Here's how the part is built. I have some questions about the finished solid (model axes, mm). A direction names the side the tool comes from. Give positions to 0.01 mm unless a question says otherwise; leave off trailing zeros. Write each loop counter-clockwise with the first axis right and the second up, starting at its lowest first coordinate (ties: lowest second). Pieces come first, ordered by that corner, then holes. Notation, with made-up numbers: M 75.5,-31.75 L 101.5,-31.75 A13 ccw 101.5,-18.75 Z; hole C 81.25,5 d11. An arc over 180 degrees is marked long. Use one line per item in the form item = value. Start each with the question number.
from build123d import *
from build123d.topology import SkipClean

# Parameters (mm, degrees)
SKETCH1_R                = 1.25
BOSS_EXTRUDE1_DEPTH      = 11
BOSS_EXTRUDE2_DEPTH      = 1.25
BOSS_EXTRUDE2_DEPTH_BACK = 1.25
SKETCH2_R                = 1.75
SKETCH3_R                = 0.75
CUT_EXTRUDE2_DEPTH       = 3


with BuildPart() as part:
    # Sketch1 → Boss-Extrude1 (new body)
    with BuildSketch(Plane(origin=(0, 0, 0), x_dir=(1, 0, 0), z_dir=(0, 1, 0))):
        with Locations(Location((0, 0, 0), (0, 0, 270))):
            Circle(SKETCH1_R)
    extrude(amount=BOSS_EXTRUDE1_DEPTH)

    # Sketch2 → Boss-Extrude2 (add, two sides: drawn at the far end of the back side and taken through both)
    with SkipClean():  # the faces are left unmerged after this step: merging them gives an invalid solid
        with BuildSketch(Plane(origin=(0, 0, 0), x_dir=(0, 0, -1), z_dir=(1, 0, 0)).offset(-BOSS_EXTRUDE2_DEPTH_BACK)):
            Circle(SKETCH2_R)
        extrude(amount=BOSS_EXTRUDE2_DEPTH + BOSS_EXTRUDE2_DEPTH_BACK)

    # Sketch3 → Cut-Extrude2 (cut)
    with SkipClean():  # the faces are left unmerged after this step: merging them gives an invalid solid
        with BuildSketch(Plane(origin=(1.25, 0, 0), x_dir=(0, 0, -1), z_dir=(1, 0, 0))):
            Circle(SKETCH3_R)
        extrude(amount=-CUT_EXTRUDE2_DEPTH, mode=Mode.SUBTRACT)


solid = part.part
1) Suppose I cut it at D-D, the plane y = 7.75. List the corners of the cut face in (x, z) for me, and give its area (3 significant figures).
2) Suppose I cut it at C-C, the plane z = -1.4. List the corners of the cut face in (x, y) for me.
3) Suppose I cut it at A-A, the plane x = 0. List the corners of the cut face in (y, z) for me.
4) Please list where these lines run through material, in increasing order: line 1 (Z direction, x = -0.05, y = 0); line 2 (Y direction, x = 0, z = 0); line 3 (Z direction, x = -1, y = 7).
5) Thinking about a two-plate mould opening in Y: for faces 1 (the face through (0, 11, 0)), 2 (the face through (1.25, -1, 0)), 3 (the face through (0.02, 0.03, 0.75)), which applies, released by +Y, released by -Y, zero draft, split by the parting line, or undercut?
6) Suppose I cut it at B-B, the plane y = 0.5. List the corners of the cut face in (x, z) for me, and give its area (3 significant figures).
7) On a 3-axis mill with a long thin cutter (end or side, diameter ignored), from which of +Z, -Z, +X, -X, +Y, -Y can I reach the whole of each face in a straight line? I mean faces 4 (the face through (-1.25, -1, 0)), 5 (the face through (0.38, 6.04, 1.19)). Say none if no direction works.
8) Will this pin go through, and if not, where does the flat tip stop? P1, Ø1, axis at x = 0.5, y = 3.5, coming from the -Z side.
Checks:
q1.outline = C 0,0 d2.5
q1.area = 4.91 mm^2
q2.outline = M -1.25,-1.05 L 1.25,-1.05 L 1.25,1.05 L -1.25,1.05 Z
q3.outline = M 1.22,-1.25 L 11,-1.25 L 11,1.25 L 1.22,1.25 A1.75 ccw long Z; hole C 0,0 d1.5
q4.line_1 = -1.75 to -0.75, 0.75 to 1.75
q4.line_2 = -1.75 to -0.75, 0.75 to 11
q4.line_3 = -0.75 to 0.75
q5.face_1 = released by +Y
q5.face_2 = zero draft
q5.face_3 = undercut
q6.outline = M -1.25,-1.68 L 1.25,-1.68 L 1.25,-0.56 L -1.25,-0.56 Z; M -1.25,0.56 L 1.25,0.56 L 1.25,1.68 L -1.25,1.68 Z
q6.area = 5.59 mm^2
q7.face_4 = +Z, -Z, -X, +Y, -Y
q7.face_5 = +Y
q8.P1 = -1.25
